Read the model definition and answer for the solid it produces. Units are mm, in the model's axes. A direction names the side the tool comes from. Coordinates: 2 decimals unless noted, no trailing zeros. Order: outer loops, then holes, each group sorted by start corner. A loop starts at its lowest first (then second) coordinate and runs counter-clockwise, first axis right, second up.
Autodesk Inventor part; units mm, degrees
ref_plane "YZ Plane" through (0, 0, 0) normal (1, 0, 0) x (0, 1, 0)
ref_plane "XZ Plane" through (0, 0, 0) normal (0, 1, 0) x (-1, 0, 0)
ref_plane "XY Plane" through (0, 0, 0) normal (0, 0, 1) x (1, 0, 0)
sketch "スケッチ1" plane through (0, 0, 0) normal (0, 0, 1) x (1, 0, 0)
  line L0 (7.5, 7.5) -> (-7.5, 7.5)
  line L1 (-7.5, 7.5) -> (-7.5, -7.5)
  line L2 (-7.5, -7.5) -> (7.5, -7.5)
  line L3 (7.5, -7.5) -> (7.5, 7.5)
  line L4 (7.5, 7.5) -> (-7.5, -7.5) construction
  line L5 (-7.5, 7.5) -> (7.5, -7.5) construction
  line L6 (-6.5, 6.5) -> (6.5, 6.5)
  line L7 (6.5, 6.5) -> (6.5, -6.5)
  line L8 (6.5, -6.5) -> (-6.5, -6.5)
  line L9 (-6.5, -6.5) -> (-6.5, 6.5)
  point P0 (0, 0)
  dimension "d0" = 15
  dimension "d1" = 15
  dimension "d2" = 1
extrude "押し出し1" add sketch "スケッチ1" along normal blind 300
sketch "スケッチ2" plane through (-7.5, 7.5, 0) normal (0, 1, 0) x (1, 0, 0)
  circle A0 centre (7.5, -10) radius 1.6
  circle A1 centre (7.5, -20) radius 1.6
  circle A2 centre (7.5, -30) radius 1.6
  circle A3 centre (7.5, -290) radius 1.6
  circle A4 centre (7.5, -280) radius 1.6
  circle A5 centre (7.5, -270) radius 1.6
  line L0 (15, -300) -> (0, -300)
  line L1 (15, 0) -> (0, 0)
  point P0 (7.5, 0)
  point P1 (7.5, 0)
  dimension "d5" = 3.2
  dimension "d6" = 3.2
  dimension "d7" = 3.2
  dimension "d8" = 3.2
  dimension "d9" = 3.2
  dimension "d10" = 3.2
  dimension "d11" = 10
  dimension "d12" = 10
  dimension "d13" = 10
  dimension "d14" = 10
  dimension "d15" = 10
  dimension "d16" = 10
extrude "押し出し2" cut sketch "スケッチ2" against normal through all
properties part number "オムニ_角柱9" material "アルミニウム 6061"
1) A cutting plane is placed at B-B, the plane z = 110. Determine the outline of the cut face in (x, y), and give its area (3 significant figures).
A:
outline: (-7.5, -7.5) - (7.5, -7.5) - (7.5, 7.5) - (-7.5, 7.5) - close; hole (-6.5, -6.5) - (6.5, -6.5) - (6.5, 6.5) - (-6.5, 6.5) - close
area: 56.0 mm2
2) A cutting plane is placed at A-A, the plane y = 1. Determine the outline of the cut face in (x, z).
A:
outline: (-7.5, 0) - (-6.5, 0) - (-6.5, 300) - (-7.5, 300) - close; (6.5, 0) - (7.5, 0) - (7.5, 300) - (6.5, 300) - close
3) Straight lines are drawn through the part: line 1 (Y direction, x = 5.75, z = 279.5); line 2 (X direction, y = -6.65, z = 280). For each, find the intervals that lie inside material, in ascending order.
A:
line 1: y = -7.5 to -6.5, 6.5 to 7.5
line 2: x = -7.5 to -1.6, 1.6 to 7.5
4) A flat-ended cylindrical pin translates along its axis: pin 1 Ø5 at (x, z) = (0, 20) entering from +Y. Find the tip coordinate at first contact, or state that the pin passes through.
A:
pin 1: stops at y = 7.5
5) Which of the six approach directions +Z, -Z, +X, -X, +Y, -Y give full straight-line access (tool end or side, diameter ignored) to faces 5 (the flat face through (0, -6.5, 148)), 6 (the flat face through (-7.5, 0, 148))?
A:
face 5: +Z, -Z
face 6: +Z, -Z, -X, +Y, -Y
6) Determine the mould class of faces 1 (the flat face through (0, 7.5, 148)), 2 (the flat face through (6.5, 0, 148)), 3 (the flat face through (7.5, 0, 148)), 4 (the flat face through (-6.5, 0, 148)) for opening direction X: pulls with the +X half, pulls with the -X half, needs draft (parallel to the pull), parting line crosses it, or undercut.
A:
face 1: needs draft
face 2: undercut
face 3: pulls with the +X half
face 4: undercut
